The listing builds one solid part. Answer for the finished solid, in the listing's coordinates (mm). A direction names the side the tool comes from. Round coordinates to 2 decimals unless told otherwise and drop trailing zeros. Write each loop counter-clockwise with the first axis right and the second up, starting at its lowest first coordinate (ties: lowest second). Pieces come first, ordered by that corner, then holes. Notation, with made-up numbers: (-11, -3) - (-1, -3) arc R33 ccw to (-1, 28) - close; hole circle Ø9 at (-5, 70.5). An arc over 180 degrees is marked (long way). Return JSON: item names as keys, results as strings. Group by question number.
(1) Section C-C, the plane y = 20 is taken. Write down the section's boundary in (x, z).
(2) Section B-B, the plane z = 31.5 is taken. Write down the section's boundary in (x, y), then the cut area to 3 significant figures.
(3) This flat-tipped pin is pushed along its axis until it touches: pin 1 (10 mm diameter, centred on x = 59.5, z = 69.5, fed in from +Y). Where does it stop, or does it pass through?
(4) Section D-D, the plane x = 12.9 is taken. Write down the section's boundary in (y, z).
(5) Which of the six approach directions +Z, -Z, +X, -X, +Y, -Y give full straight-line access (tool end or side, diameter ignored) to faces 1 (the flat face through (15, 65, 14)), 2 (the cylindrical face through (2.5, 20.1, 121.4))?
(6) Determine the mould class of faces 3 (the flat face through (69, 55, 147)), 4 (the flat face through (74, 27, 0)), 5 (the cylindrical face through (2.47, 18.89, 28.82)) for opening direction Y: +Y half, -Y half, draft (parallel to the pull), parting line (faces both ways), or undercut.
(7) Find the intervals of material crossed by line 1 along Z through (x, y) = (148.25, 20); line 2 along Y through (x, z) = (148.3, 31.5); line 3 along X through (y, z) = (25, 100), in increasing order. Write a range as [from, to].
(8) Section A-A, the plane y = 35 is taken. Write down the section's boundary in (x, z), then the cut area to 3 significant figures.
```python
from build123d import *

# Parameters (mm, degrees)
SKETCH1_W               = 150
SKETCH1_H               = 150
SKETCH1_W_2             = 140
SKETCH1_H_2             = 140
BOSS_EXTRUDE1_DEPTH     = 55
SKETCH1_3_W             = 140
SKETCH1_3_H             = 140
SKETCH1_3_R             = 4
BOSS_EXTRUDE2_DEPTH     = 10
SKETCH1_4_R             = 4
SKETCH1_4_R_2           = 2
BOSS_EXTRUDE3_DEPTH     = 65
SKETCH1_5_R             = 2
BOSS_EXTRUDE4_DEPTH     = 80
CUT_EXTRUDE3_DEPTH      = 227.715680975
CUT_EXTRUDE3_DEPTH_BACK = 130
SKETCH3_R               = 2.9


with BuildPart() as part:
    # Sketch1 → Boss-Extrude1 (new body)
    with BuildSketch(Plane(origin=(0, 0, 0), x_dir=(1, 0, 0), z_dir=(0, 1, 0))):
        with Locations((75, -75)):
            Rectangle(SKETCH1_W, SKETCH1_H)
        with Locations((75, -75)):
            Rectangle(SKETCH1_W_2, SKETCH1_H_2, mode=Mode.SUBTRACT)
    extrude(amount=BOSS_EXTRUDE1_DEPTH)

    # Sketch1_3 → Boss-Extrude2 (add)
    with BuildSketch(Plane(origin=(0, 0, 0), x_dir=(1, 0, 0), z_dir=(0, 1, 0))):
        with Locations((75, -75)):
            Rectangle(SKETCH1_3_W, SKETCH1_3_H)
        with Locations(Location((12.9, -137.1, 0), (0, 0, 270))):
            Circle(SKETCH1_3_R, mode=Mode.SUBTRACT)
        with Locations(Location((137.1, -137.1, 0), (0, 0, 270))):
            Circle(SKETCH1_3_R, mode=Mode.SUBTRACT)
        with Locations(Location((137.1, -12.9, 0), (0, 0, 270))):
            Circle(SKETCH1_3_R, mode=Mode.SUBTRACT)
        with Locations(Location((12.9, -12.9, 0), (0, 0, 270))):
            Circle(SKETCH1_3_R, mode=Mode.SUBTRACT)
    extrude(amount=BOSS_EXTRUDE2_DEPTH)

    # Sketch1_4 → Boss-Extrude3 (add)
    # profile 1 of 4: a face of its own
    with BuildSketch(Plane(origin=(0, 0, 0), x_dir=(1, 0, 0), z_dir=(0, 1, 0))):
        with Locations(Location((12.9, -12.9, 0), (0, 0, 270))):
            Circle(SKETCH1_4_R)
        with Locations(Location((12.9, -12.9, 0), (0, 0, 270))):
            Circle(SKETCH1_4_R_2, mode=Mode.SUBTRACT)
    # profile 2 of 4: a face of its own
    with BuildSketch(Plane(origin=(0, 0, 0), x_dir=(1, 0, 0), z_dir=(0, 1, 0))):
        with Locations(Location((137.1, -12.9, 0), (0, 0, 270))):
            Circle(SKETCH1_4_R)
        with Locations(Location((137.1, -12.9, 0), (0, 0, 270))):
            Circle(SKETCH1_4_R_2, mode=Mode.SUBTRACT)
    # profile 3 of 4: a face of its own
    with BuildSketch(Plane(origin=(0, 0, 0), x_dir=(1, 0, 0), z_dir=(0, 1, 0))):
        with Locations(Location((137.1, -137.1, 0), (0, 0, 270))):
            Circle(SKETCH1_4_R)
        with Locations(Location((137.1, -137.1, 0), (0, 0, 270))):
            Circle(SKETCH1_4_R_2, mode=Mode.SUBTRACT)
    # profile 4 of 4: a face of its own
    with BuildSketch(Plane(origin=(0, 0, 0), x_dir=(1, 0, 0), z_dir=(0, 1, 0))):
        with Locations(Location((12.9, -137.1, 0), (0, 0, 270))):
            Circle(SKETCH1_4_R)
        with Locations(Location((12.9, -137.1, 0), (0, 0, 270))):
            Circle(SKETCH1_4_R_2, mode=Mode.SUBTRACT)
    extrude(amount=BOSS_EXTRUDE3_DEPTH)

    # Sketch1_5 → Boss-Extrude4 (add)
    with BuildSketch(Plane(origin=(0, 0, 0), x_dir=(1, 0, 0), z_dir=(0, 1, 0))):
        with Locations(Location((12.9, -137.1, 0), (0, 0, 270))):
            Circle(SKETCH1_5_R)
        with Locations(Location((137.1, -137.1, 0), (0, 0, 270))):
            Circle(SKETCH1_5_R)
        with Locations(Location((137.1, -12.9, 0), (0, 0, 270))):
            Circle(SKETCH1_5_R)
        with Locations(Location((12.9, -12.9, 0), (0, 0, 270))):
            Circle(SKETCH1_5_R)
    extrude(amount=BOSS_EXTRUDE4_DEPTH)

    # Sketch3 → Cut-Extrude3 (cut, two sides: drawn at the far end of the back side and taken through both)
    with BuildSketch(Plane(origin=(0, 0, 0), x_dir=(0, 0, -1), z_dir=(1, 0, 0)).offset(-CUT_EXTRUDE3_DEPTH_BACK)):
        with Locations((-31.5, 20)):
            Circle(SKETCH3_R)
        with Locations((-118.5, 20)):
            Circle(SKETCH3_R)
    extrude(amount=CUT_EXTRUDE3_DEPTH + CUT_EXTRUDE3_DEPTH_BACK, mode=Mode.SUBTRACT)


solid = part.part
```
Working result:
{
 "1": {"outline": "(0, 0) - (150, 0) - (150, 28.6) - (145, 28.6) - (145, 5) - (5, 5) - (5, 28.6) - (0, 28.6) - close; (0, 34.4) - (5, 34.4) - (5, 115.6) - (0, 115.6) - close; (0, 121.4) - (5, 121.4) - (5, 145) - (145, 145) - (145, 121.4) - (150, 121.4) - (150, 150) - (0, 150) - close; circle Ø8 at (12.9, 12.9); circle Ø8 at (12.9, 137.1); circle Ø8 at (137.1, 12.9); circle Ø8 at (137.1, 137.1); (145, 34.4) - (150, 34.4) - (150, 115.6) - (145, 115.6) - close"},
 "2": {"outline": "(0, 0) - (150, 0) - (150, 17.1) - (145, 17.1) - (145, 10) - (5, 10) - (5, 17.1) - (0, 17.1) - close; (0, 22.9) - (5, 22.9) - (5, 55) - (0, 55) - close; (145, 22.9) - (150, 22.9) - (150, 55) - (145, 55) - close", "area": "1,890 mm^2"},
 "3": {"pin 1": "stops at y = 10"},
 "4": {"outline": "(0, 0) - (55, 0) - (55, 5) - (10, 5) - (10, 8.9) - (65, 8.9) - (65, 10.9) - (80, 10.9) - (80, 14.9) - (65, 14.9) - (65, 16.9) - (10, 16.9) - (10, 133.1) - (65, 133.1) - (65, 135.1) - (80, 135.1) - (80, 139.1) - (65, 139.1) - (65, 141.1) - (10, 141.1) - (10, 145) - (55, 145) - (55, 150) - (0, 150) - close"},
 "5": {"face 1": "+Y", "face 2": "+X, -X"},
 "6": {"face 3": "+Y half", "face 4": "draft", "face 5": "undercut"},
 "7": {"line 1": "z = [0, 28.6], [34.4, 115.6], [121.4, 150]", "line 2": "y = [0, 17.1], [22.9, 55]", "line 3": "x = [0, 5], [145, 150]"},
 "8": {"outline": "(0, 0) - (150, 0) - (150, 150) - (0, 150) - close; circle Ø8 at (12.9, 12.9); circle Ø8 at (12.9, 137.1); circle Ø8 at (137.1, 12.9); circle Ø8 at (137.1, 137.1); hole (5, 5) - (145, 5) - (145, 145) - (5, 145) - close", "area": "3,100 mm^2"}
}
